Check sheet for the modelled part. Datum: model origin and axes. Units: mm. A direction names the side the tool comes from. Give positions to 0.01 mm unless a question says otherwise; leave off trailing zeros. Write each loop counter-clockwise with the first axis right and the second up, starting at its lowest first coordinate (ties: lowest second). Pieces come first, ordered by that corner, then holes. Notation, with made-up numbers: M 13,-35.75 L 69,-35.75 A23 cw 69,-18.75 Z; hole C 27.5,81 d9. An arc over 180 degrees is marked long. Write item = value, one per line. Start each with the question number.
1) Sectioned sample at D-D, the plane z = -34.5. Record the cut outline in (x, y), then the cut area to 3 significant figures.
2) Scan lines: L1, parallel to X at y = -0.25, z = 30; L2, parallel to Z at x = 2.5, y = -0.5. Record each from-to range of solid material in increasing order.
3) Set-up check for faces 1 (the face through (0, 0, -40.284)), 2 (the face through (-2.374, 0.748, -36.074)), 3 (the face through (0, 2, -32)): record each of +Z, -Z, +X, -X, +Y, -Y from which the full face is reachable in a straight line by a thin tool's end or side.
4) Gauge pin test, flat ends, axial feed: pin 1 (2 mm diameter, centred on y = 1.5, z = 17.5, fed in from +X); pin 2 (2 mm diameter, centred on y = 2, z = 28.5, fed in from +X). Record the tip position at first contact, or that the pin passes through.
5) Sectioned sample at A-A, the plane x = 0. Record the cut outline in (y, z) (3 decimals), then the cut area to 3 significant figures.
6) Sectioned sample at C-C, the plane z = -6.5. Record the cut outline in (x, y) (3 decimals).
7) Draft check along Z on faces 4 (the face through (0, 0, 39.395)), 5 (the face through (-0.69, 3.1, 3.26)), 6 (the face through (1, -2, -31.255)). Enter one of: pulls with the +Z half, pulls with the -Z half, needs draft (parallel to the pull), parting line crosses it, or undercut.
Autodesk Inventor part; units mm, degrees
sketch "Sketch1" plane through (0, 0, 0) normal (0, 0, 1) x (1, 0, 0)
  circle A0 centre (0, 0) radius 3.175
  dimension "d0" = 6.35
extrude "Extrusion1" add sketch "Sketch1" along normal blind 39.3954 and the other way blind 40.2844
ref_plane "Work Plane1" through (0, 0, -31.8262) normal (0, 0, 1) x (1, 0, 0)
sketch "Sketch2" plane through (0, 0, -31.8262) normal (0, 0, 1) x (1, 0, 0)
  circle A0 centre (0, 0) radius 2
  circle A1 centre (0, 0) radius 3.27
  dimension "d9" = 4
  dimension "d10" = 1.27
extrude "Extrusion2" cut sketch "Sketch2" along normal mid plane 1.143
sketch "Sketch3" plane through (0, 0, -40.2844) normal (0, 0, -1) x (-1, 0, 0)
  circle A0 centre (0, 0) radius 3.175
  circle A1 centre (0, 0) radius 3.175
  circle A2 centre (0, 0) radius 2.4892
  dimension "d13" = 4.9784
  dimension "d14" = 0
extrude "Extrusion3" cut sketch "Sketch3" against normal up to next
chamfer "Chamfer1" distance 0.635 angle 45 2 edges at (-3.175, 0, 39.3954) (2.4892, 0, -40.2844)
properties part number "J005526" material "ALUMINUM, 2024-T4/T351"
Data:
q1.outline = C 0,0 d4.98
q1.area = 19.5 mm2
q2.L1 = -3.17 to 3.17
q2.L2 = -31.25 to 39.39
q3.face_1 = -Z, +X, -X, +Y, -Y
q3.face_2 = -Z
q3.face_3 = none
q4.pin_1 = 3.14
q4.pin_2 = 3.01
q5.outline = M -3.175,-31.255 L -2,-31.255 L -2,-32.398 L -2.489,-32.398 L -2.489,-39.649 L -1.854,-40.284 L 1.854,-40.284 L 2.489,-39.649 L 2.489,-32.398 L 2,-32.398 L 2,-31.255 L 3.175,-31.255 L 3.175,38.76 L 2.54,39.395 L -2.54,39.395 L -3.175,38.76 Z
q5.area = 492 mm2
q6.outline = C 0,0 d6.35
q7.face_4 = pulls with the +Z half
q7.face_5 = needs draft
q7.face_6 = undercut
